Input: part model. Units: mm. Frame: model coordinates. Face numbers are marked on the shaded views. A direction names the side the tool comes from. Give positions to 0.01 mm unless a question says otherwise; leave off trailing zeros. Loops run counter-clockwise (first coordinate to the right, second up) from the corner with the lowest first, then second, coordinate; pieces in that order, holes last. Notation, with made-up numbers: (-6, 0) -> (28, 0) arc R27 cw to (28, 34) -> close; hole circle Ø9 at (58, 19.5). An arc over 180 degrees is marked (long way). Use CSV: the item, a comma, the result in double quotes.
```python
from build123d import *

# Parameters (mm, degrees)
F0_W     = 126
F0_H     = 73
F1_DEPTH = 2
F2_W     = 1.7
F2_H     = 1.5
F2_W_2   = 19.1
F2_H_2   = 70
F3_DEPTH = 16
F5_DEPTH = 100
F6_R     = 0.1


with BuildPart() as f1:
    # F0 (on Top) → F1 (new body)
    with BuildSketch(Plane.XY):
        Rectangle(F0_W, F0_H)
    extrude(amount=F1_DEPTH)

    # F2 (on face) → F3 (join)
    with BuildSketch(Plane.XY.offset(2)):
        Polygon((42.4, 35), (61.5, 35), (61.5, -35), (42.4, -35), (42.4, -36.5), (63, -36.5), (63, 36.5), (42.4, 36.5), align=None)
        with Locations((41.55, 35.75)):
            Rectangle(F2_W, F2_H)
        with Locations((31.15, 35.75)):
            Rectangle(F2_W_2, F2_H)
        with Locations((41.55, -35.75)):
            Rectangle(F2_W, F2_H)
        with Locations((20.75, 35.75)):
            Rectangle(F2_W, F2_H)
        with Locations((31.15, -35.75)):
            Rectangle(F2_W_2, F2_H)
        with Locations((10.35, 35.75)):
            Rectangle(F2_W_2, F2_H)
        with Locations((20.75, -35.75)):
            Rectangle(F2_W, F2_H)
        with Locations((-0.05, 35.75)):
            Rectangle(F2_W, F2_H)
        with Locations((10.35, -35.75)):
            Rectangle(F2_W_2, F2_H)
        with Locations((-10.45, 35.75)):
            Rectangle(F2_W_2, F2_H)
        with Locations((-0.05, -35.75)):
            Rectangle(F2_W, F2_H)
        with Locations((-20.85, 35.75)):
            Rectangle(F2_W, F2_H)
        with Locations((-10.45, -35.75)):
            Rectangle(F2_W_2, F2_H)
        with Locations((-31.25, 35.75)):
            Rectangle(F2_W_2, F2_H)
        with Locations((-20.85, -35.75)):
            Rectangle(F2_W, F2_H)
        with Locations((-41.65, 35.75)):
            Rectangle(F2_W, F2_H)
        with Locations((-31.25, -35.75)):
            Rectangle(F2_W_2, F2_H)
        Polygon((-61.5, 35), (-42.5, 35), (-42.5, 36.5), (-63, 36.5), (-63, -36.5), (-42.5, -36.5), (-42.5, -35), (-61.5, -35), align=None)
        with Locations((-41.65, -35.75)):
            Rectangle(F2_W, F2_H)
        with Locations((-41.65, 0)):
            Rectangle(F2_W, F2_H_2)
        with Locations((-20.85, 0)):
            Rectangle(F2_W, F2_H_2)
        with Locations((-0.05, 0)):
            Rectangle(F2_W, F2_H_2)
        with Locations((20.75, 0)):
            Rectangle(F2_W, F2_H_2)
        with Locations((41.55, 0)):
            Rectangle(F2_W, F2_H_2)
    extrude(amount=F3_DEPTH)

    # F4 (on face) → F5 (cut)
    with BuildSketch(Plane.XZ.offset(36.5)):
        with BuildLine():
            ThreePointArc((-49.5, 9), (-52, 11.5), (-54.5, 9))
            Line((-54.5, 9), (-49.5, 9))
        make_face()
        with BuildLine():
            ThreePointArc((54.5, 9), (52, 11.5), (49.5, 9))
            Line((49.5, 9), (54.5, 9))
        make_face()
        with BuildLine():
            Line((54.5, 9), (49.5, 9))
            ThreePointArc((49.5, 9), (52, 6.5), (54.5, 9))
        make_face()
        with BuildLine():
            ThreePointArc((33.8, 9), (31.3, 11.5), (28.8, 9))
            Line((28.8, 9), (33.8, 9))
        make_face()
        with BuildLine():
            Line((33.8, 9), (28.8, 9))
            ThreePointArc((28.8, 9), (31.3, 6.5), (33.8, 9))
        make_face()
        with BuildLine():
            ThreePointArc((13.1, 9), (10.6, 11.5), (8.1, 9))
            Line((8.1, 9), (13.1, 9))
        make_face()
        with BuildLine():
            Line((13.1, 9), (8.1, 9))
            ThreePointArc((8.1, 9), (10.6, 6.5), (13.1, 9))
        make_face()
        with BuildLine():
            ThreePointArc((-8.1, 9), (-10.6, 11.5), (-13.1, 9))
            Line((-13.1, 9), (-8.1, 9))
        make_face()
        with BuildLine():
            Line((-8.1, 9), (-13.1, 9))
            ThreePointArc((-13.1, 9), (-10.6, 6.5), (-8.1, 9))
        make_face()
        with BuildLine():
            ThreePointArc((-28.8, 9), (-31.3, 11.5), (-33.8, 9))
            Line((-33.8, 9), (-28.8, 9))
        make_face()
        with BuildLine():
            Line((-28.8, 9), (-33.8, 9))
            ThreePointArc((-33.8, 9), (-31.3, 6.5), (-28.8, 9))
        make_face()
        with BuildLine():
            Line((-49.5, 9), (-54.5, 9))
            ThreePointArc((-54.5, 9), (-52, 6.5), (-49.5, 9))
        make_face()
    extrude(amount=-F5_DEPTH, mode=Mode.SUBTRACT)

    # F6
    f6_edges = [f1.edges().sort_by_distance(p)[0] for p in [
        (-63, -36.5, 9),
        (63, -36.5, 9),
        (63, 36.5, 9),
        (-63, 36.5, 9),
    ]]
    fillet(f6_edges, radius=F6_R)


solid = f1.part
```
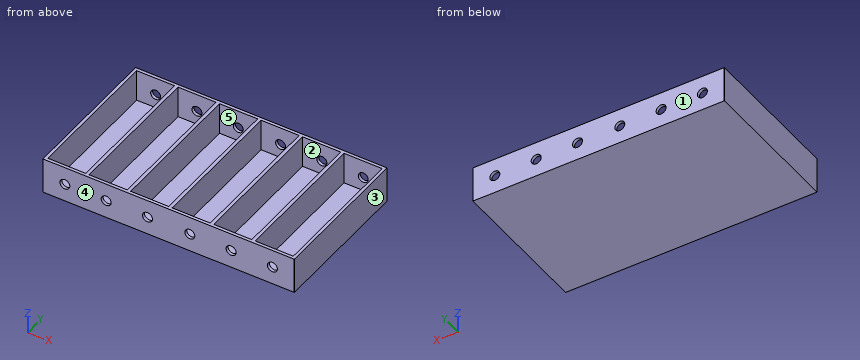
1) Section query B-B (z = 15). Give the number of separate pieces and of enclosed holes in the cut face, then the cut area to 3 significant figures.
From the geometry:
separate pieces,"1"
enclosed holes,"6"
area,"1,180 mm^2"
2) Section query C-C (y = -25). Return loops of the section in (x, z).
From the geometry:
outline,"(-63, 0) -> (63, 0) -> (63, 18) -> (61.5, 18) -> (61.5, 2) -> (42.4, 2) -> (42.4, 18) -> (40.7, 18) -> (40.7, 2) -> (21.6, 2) -> (21.6, 18) -> (19.9, 18) -> (19.9, 2) -> (0.8, 2) -> (0.8, 18) -> (-0.9, 18) -> (-0.9, 2) -> (-20, 2) -> (-20, 18) -> (-21.7, 18) -> (-21.7, 2) -> (-40.8, 2) -> (-40.8, 18) -> (-42.5, 18) -> (-42.5, 2) -> (-61.5, 2) -> (-61.5, 18) -> (-63, 18) -> close"
3) Reachability of the marked faces 1 and 2 from +Z, -Z, +X, -X, +Y, -Y: full face, straight path, thin tool, end or side. Return the list, or none.
From the geometry:
face 1,"+Z, -Z, +X, -X, +Y"
face 2,"+Z"
4) Ray query, line 1 (Y direction, x = -39.5, z = 8.25); line 2 (Z direction, x = 52, y = -35.5); line 3 (Z direction, x = 11.5, y = 23.5). Return the intervals inside material, ascending.
From the geometry:
line 1,"y = -36.5 to -35, 35 to 36.5"
line 2,"z = 0 to 6.5, 11.5 to 18"
line 3,"z = 0 to 2"
5) Section query D-D (x = -5.5). Return loops of the section in (y, z), then the cut area to 3 significant figures.
From the geometry:
outline,"(-36.5, 0) -> (36.5, 0) -> (36.5, 18) -> (35, 18) -> (35, 2) -> (-35, 2) -> (-35, 18) -> (-36.5, 18) -> close"
area,"194 mm^2"
6) Section query A-A (x = 10.6). Return loops of the section in (y, z).
From the geometry:
outline,"(-36.5, 0) -> (36.5, 0) -> (36.5, 6.5) -> (35, 6.5) -> (35, 2) -> (-35, 2) -> (-35, 6.5) -> (-36.5, 6.5) -> close; (-36.5, 11.5) -> (-35, 11.5) -> (-35, 18) -> (-36.5, 18) -> close; (35, 11.5) -> (36.5, 11.5) -> (36.5, 18) -> (35, 18) -> close"
7) Contact query for flat-ended pins moving along their axis: pin 1 (15.5 mm diameter, centred on x = 9, y = 13.5, fed in from +Z); pin 2 (4 mm diameter, centred on x = 10.6, z = 9, fed in from -Y). Output: stop coordinate, or through.
From the geometry:
pin 1,"stops at z = 2"
pin 2,"passes through"
8) Mould query, pull axis X, two halves, no side actions, for the marked faces 3, 4 and 5. Classes: pulls with the +X half, pulls with the -X half, needs draft (parallel to the pull), parting line crosses it, or undercut.
From the geometry:
face 3,"pulls with the +X half"
face 4,"needs draft"
face 5,"undercut"
